Verification items for this drawing (mm, ordinates from the low corner). A direction names the side the tool comes from. Coordinates: 2 decimals unless noted, no trailing zeros. Order: outer loops, then holes, each group sorted by start corner. A loop starts at its lowest first (then second) coordinate and runs counter-clockwise, first axis right, second up. Notation, with made-up numbers: M -22.5,66 L 17.5,66 A24 cw 17.5,105 Z; hole C 52.25,27.5 d9. An arc over 180 degrees is marked long. One line per item, written item: value. Start each with the question number.
1) Sectioned sample at B-B, the plane y = 1.5. Enter the section's corners in (x, z), then the cut area to 3 significant figures.
2) Sectioned sample at A-A, the plane x = 8. Enter the section's corners in (y, z).
3) Thickness scan on L1, parallel to X at y = 1.65, z = 12; L2, parallel to Z at x = 8.5, y = 2.65; L3, parallel to Z at x = 9.5, y = 2.8 (1 decimal). Record the ranges inside material, lowest first. Write a range as from..to.
4) Access from +Z, -Z, +X, -X, +Y, -Y to the whole of each face (thin tool, end or side, straight path). Record for the marked faces 1, 2 and 3.
5) Go/stop test with a flat-tipped pin: P1, Ø1.5, axis at x = 6.5, y = 2, coming from the +Z side. Record where the tip stops, or that it passes through.
6) Draft check along Z on the marked faces 4, 5, 6 and 7. Enter one of: pulls with the +Z half, pulls with the -Z half, needs draft (parallel to the pull), parting line crosses it, or undercut.
7) Sectioned sample at D-D, the plane x = 1. Enter the section's corners in (y, z).
8) Sectioned sample at C-C, the plane z = 5.75. Enter the section's corners in (x, y).
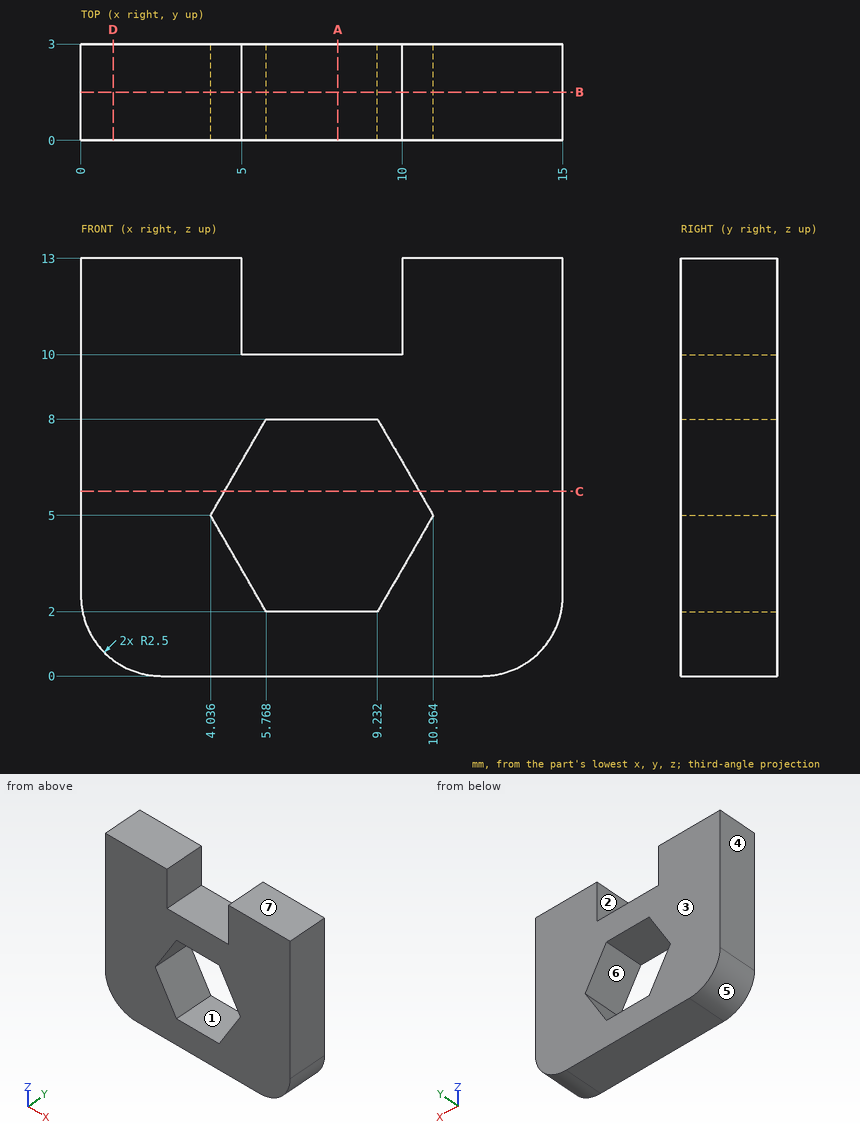
Final values:
1. outline: M 0,2.5 A2.5 ccw 2.5,0 L 12.5,0 A2.5 ccw 15,2.5 L 15,13 L 10,13 L 10,10 L 5,10 L 5,13 L 0,13 Z; hole M 4.04,5 L 5.77,2 L 9.23,2 L 10.96,5 L 9.23,8 L 5.77,8 Z
1. area: 146 mm^2
2. outline: M 0,0 L 3,0 L 3,2 L 0,2 Z; M 0,8 L 3,8 L 3,10 L 0,10 Z
3. L1: x = 0..5, 10..15
3. L2: z = 0..2, 8..10
3. L3: z = 0..2.5, 7.5..10
4. face 1: +Y, -Y
4. face 2: +Z, +Y, -Y
4. face 3: +Z, -Z, +X, -X, +Y
5. P1: stops at z = 10
6. face 4: needs draft
6. face 5: pulls with the -Z half
6. face 6: undercut
6. face 7: pulls with the +Z half
7. outline: M 0,0.5 L 3,0.5 L 3,13 L 0,13 Z
8. outline: M 0,0 L 4.47,0 L 4.47,3 L 0,3 Z; M 10.53,0 L 15,0 L 15,3 L 10.53,3 Z
